```python
from build123d import *

# Parameters (mm, degrees)
SKETCH_R        = 3.5
SKETCH_R_2      = 1.6
PAD_DEPTH       = 1.4
SKETCH001_W     = 119.586
SKETCH001_H     = 17.78
SKETCH001_R     = 1.6
PAD001_DEPTH    = 1.5
SKETCH002_R     = 3.5
SKETCH002_R_2   = 1.6
PAD002_DEPTH    = 1.4
SKETCH003_R     = 1.6
POCKET_DEPTH    = 2.901
PAD003_DEPTH    = 17.78
CHAMFER_SIZE    = 2.2
CHAMFER002_SIZE = 0.6
SKETCH014_W     = 2
SKETCH014_H     = 1.4
SKETCH014_W_2   = 1.5
PAD009_DEPTH    = 85
SKETCH016_W     = 27.172
SKETCH016_H     = 2
PAD010_DEPTH    = 1.4


with BuildPart() as part:
    # Sketch (on Face1 of CopyPcb_f5c5) → Pad (new body)
    with BuildSketch(Plane(origin=(-93.484762, 101.426, -1.6), x_dir=(1, 0, 0), z_dir=(0, 0, -1))):
        with Locations((113.233762, 92.79)):
            Circle(SKETCH_R)
        with Locations((113.233762, 92.79)):
            Circle(SKETCH_R_2, mode=Mode.SUBTRACT)
    extrude(amount=PAD_DEPTH)

    # Sketch001 (on Face4 of Pad) → Pad001 (join)
    with BuildSketch(Plane(origin=(-93.484762, 101.426, -3), x_dir=(1, 0, 0), z_dir=(0, 0, -1))):
        with Locations((153.277762, 92.79)):
            Rectangle(SKETCH001_W, SKETCH001_H)
        with Locations((113.233762, 92.79)):
            Circle(SKETCH001_R, mode=Mode.SUBTRACT)
    extrude(amount=PAD001_DEPTH)

    # Sketch002 (on Face3 of Pad001) → Pad002 (join)
    with BuildSketch(Plane(origin=(-93.484762, 101.426, -3), x_dir=(1, 0, 0), z_dir=(0, 0, 1))):
        with Locations((160.733762, -92.79)):
            Circle(SKETCH002_R)
        with Locations((160.733762, -92.79)):
            Circle(SKETCH002_R_2, mode=Mode.SUBTRACT)
    extrude(amount=PAD002_DEPTH)

    # Sketch003 (on Face11 of Pad002) → Pocket (cut, through all)
    with BuildSketch(Plane(origin=(-93.484762, 101.426, -4.5), x_dir=(1, 0, 0), z_dir=(0, 0, -1))):
        with Locations((160.733762, 92.79)):
            Circle(SKETCH003_R)
    extrude(amount=-POCKET_DEPTH, mode=Mode.SUBTRACT)

    # Sketch004 (on Face6 of Pocket) → Pad003 (join)
    with BuildSketch(Plane(origin=(-93.484762, -0.254, -1.6), x_dir=(1, 0, 0), z_dir=(0, -1, 0))):
        with BuildLine():
            Line((202.656762, -1.4), (205.656762, 1.6))
            Line((205.656762, 1.6), (213.070762, 1.6))
            Line((213.070762, 1.3), (213.070762, 1.6))
            ThreePointArc((213.070762, 1.3), (211.870762, 0.1), (213.070762, -1.1))
            Line((213.070762, -1.1), (213.070762, -1.4))
            Line((213.070762, -1.4), (202.656762, -1.4))
        make_face()
    extrude(amount=-PAD003_DEPTH)

    # Chamfer
    chamfer_edges = [part.edges().sort_by_distance(p)[0] for p in [
        (18.149, 8.636, -4.5),
        (65.649, 8.636, -4.5),
    ]]
    chamfer(chamfer_edges, length=CHAMFER_SIZE)

    # Chamfer002
    chamfer002_edges = [part.edges().sort_by_distance(p)[0] for p in [
        (16.249, 8.636, -3),
        (63.749, 8.636, -3),
    ]]
    chamfer(chamfer002_edges, length=CHAMFER002_SIZE)

    # Sketch014 (on Face7 of Chamfer002) → Pad009 (join)
    with BuildSketch(Plane(origin=(0, 101.426, -1.6), x_dir=(0, -1, 0), z_dir=(-1, 0, 0))):
        with Locations((84.9, -0.7)):
            Rectangle(SKETCH014_W, SKETCH014_H)
        with Locations((100.93, -0.7)):
            Rectangle(SKETCH014_W_2, SKETCH014_H)
    extrude(amount=-PAD009_DEPTH)

    # Sketch016 (on Face4 of Pad009) → Pad010 (join)
    with BuildSketch(Plane(origin=(-93.484762, 101.426, -3), x_dir=(1, 0, 0), z_dir=(0, 0, 1))):
        with Locations((192.070762, -93.04)):
            Rectangle(SKETCH016_W, SKETCH016_H)
    extrude(amount=PAD010_DEPTH)


solid = part.part
```
CAD build for the part. Positions are in the model's coordinates, mm. A direction names the side the tool comes from. Give positions to 0.01 mm unless a question says otherwise; leave off trailing zeros. Write each loop counter-clockwise with the first axis right and the second up, starting at its lowest first coordinate (ties: lowest second). Pieces come first, ordered by that corner, then holes. Notation, with made-up numbers: M -28,87 L 26,87 A26 ccw 26,102 Z; hole C 1.25,-5 d4. An arc over 180 degrees is marked long. Return JSON: item names as keys, results as strings. Group by question number.
(1) 3-axis set-ups, long thin cutter, end or side, ignore diameter. For faces 5 (the face through (65.99, 7.48, -2.41)), 6 (the face through (54, 9, -3)), 7 (the face through (42, 17, -1.6)): which of +Z, -Z, +X, -X, +Y, -Y reach the whole face in a straight line?
(2) Band-saw the part on B-B (y = 14). Give the cut face in (x, z).
(3) Mould opens along X. For faces 1 (the face through (65.65, 8.57, -1.95)), 2 (the face through (59, 17.526, -3)), 3 (the face through (118.386, 8.512, -1.474)), 4 (the face through (21.38, 8.12, -2.41)) say: pulls with the +X half, pulls with the -X half, needs draft (parallel to the pull), parting line crosses it, or undercut.
(4) Band-saw the part on A-A (x = 105.5). Give the cut face in (y, z), and give its area (3 significant figures).
(5) Flat gauge pins, fed straight in: pin 1 Ø1.1 at (y, z) = (8.5, -2) entering from -X; pin 2 Ø5.5 at (x, y) = (18.5, 10) entering from +Z; pin 3 Ø1.5 at (x, z) = (103.5, -2.5) entering from +Y; pin 4 Ø0.7 at (y, z) = (0.5, -2) entering from +X. Where does each tip first touch, or does it go through?
(6) Drill centre lines: L1, parallel to X at y = 10, z = -1.75; L2, parallel to Y at x = 34, z = -1.9; L3, parallel to Z at x = 11.5, y = 6. Where is each one in solid material? Low to high. Write a range as [from, to].
Entries:
{
 "1": {"face 5": "-Z", "face 6": "+Z", "face 7": "+Z, -X, +Y, -Y"},
 "2": {"outline": "M 0,-4.5 L 119.59,-4.5 L 119.59,-2.7 A1.2 cw 119.59,-0.3 L 119.59,0 L 112.17,0 L 109.17,-3 L 0,-3 Z"},
 "3": {"face 1": "undercut", "face 2": "needs draft", "face 3": "pulls with the +X half", "face 4": "undercut"},
 "4": {"outline": "M -0.25,-4.5 L 17.53,-4.5 L 17.53,-3 L 9.39,-3 L 9.39,-1.6 L 7.39,-1.6 L 7.39,-3 L -0.25,-3 Z", "area": "29.5 mm^2"},
 "5": {"pin 1": "stops at x = 16.1", "pin 2": "stops at z = -1.6", "pin 3": "stops at y = 17.53", "pin 4": "stops at x = 118.74"},
 "6": {"L1": "x = [16.53, 18.91], [20.59, 22.97], [64.03, 66.41], [68.09, 70.47], [110.42, 118.41]", "L2": "y = [-0.25, 1.25], [15.53, 17.53]", "L3": "z = [-4.5, -3]"}
}
